```python
from build123d import *

# Parameters (mm, degrees)
F0_R     = 0.6
F1_DEPTH = 4


with BuildPart() as f1:
    # F0 (on Front) → F1 (new body)
    with BuildSketch(Plane.XZ):
        with BuildLine():
            ThreePointArc((8, 0), (9.478575, -1.518464), (10.999917, -0.042849))
            ThreePointArc((10.999917, -0.042849), (10.999979, -0.021425), (11, 0))
            ThreePointArc((11, 0), (0, 11), (-11, 0))
            ThreePointArc((-11, 0), (-1.5, 9.5), (8, 0))
        make_face()
        with Locations((9.5, 0)):
            Circle(F0_R, mode=Mode.SUBTRACT)
    extrude(amount=F1_DEPTH)


solid = f1.part
```
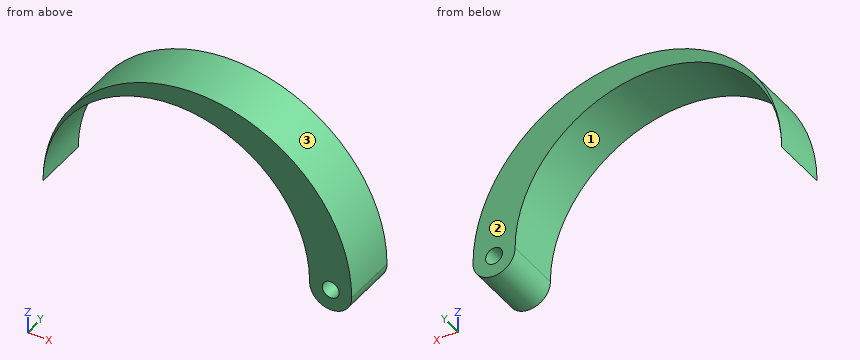
Work out the finished part from the listing and answer in its coordinate system (mm). Face numbers are marked on the shaded views. Round coordinates to 2 decimals unless told otherwise and drop trailing zeros. Order: outer loops, then holes, each group sorted by start corner. A loop starts at its lowest first (then second) coordinate and runs counter-clockwise, first axis right, second up.
Q1. A cutting plane is placed at C-C, the plane x = 9.5. Determine the outline of the cut face in (y, z), then the cut area to 3 significant figures.
Solution:
outline: (-4, -1.52) - (0, -1.52) - (0, -0.6) - (-4, -0.6) - close; (-4, 0.6) - (0, 0.6) - (0, 5.55) - (-4, 5.55) - close
area: 23.5 mm2
Q2. A cutting plane is placed at B-B, the plane y = -1.25. Determine the outline of the cut face in (x, z).
Solution:
outline: (-11, 0) arc R9.5 cw to (8, 0) arc R1.5 ccw to (11, -0.04) arc R11.19 ccw to (11, 0) arc R11 ccw to start; hole circle Ø1.2 at (9.5, 0)
Q3. A cutting plane is placed at D-D, the plane x = 2.25. Determine the outline of the cut face in (y, z).
Solution:
outline: (-4, 8.73) - (0, 8.73) - (0, 10.77) - (-4, 10.77) - close
Q4. A cutting plane is placed at A-A, the plane z = 7.25. Determine the outline of the cut face in (x, y), then the cut area to 3 significant figures.
Solution:
outline: (-8.27, -4) - (-7.64, -4) - (-7.64, 0) - (-8.27, 0) - close; (4.64, -4) - (8.27, -4) - (8.27, 0) - (4.64, 0) - close
area: 17.1 mm2
Q5. Given pin 1 Ø1.4 at (x, z) = (9.5, 0) entering from -Y; pin 2 Ø2 at (x, y) = (8, -3) entering from -Z; pin 3 Ø1.5 at (y, z) = (-2.5, 4) entering from +X; pin 4 Ø1 at (x, y) = (3, -3) entering from +Z, each flat-ended and moving along its own axis, determine where each tip first touches the part or whether it passes through.
Solution:
pin 1: stops at y = -4
pin 2: stops at z = -1.43
pin 3: stops at x = 10.51
pin 4: stops at z = 10.71
Q6. Find the intervals of material crossed by line 1 along X through (y, z) = (-0.85, 6.75); line 2 along Z through (x, y) = (9.5, -2.1); line 3 along X through (y, z) = (-0.45, 8.5), in increasing order.
Solution:
line 1: x = -8.69 to -8.18, 5.18 to 8.69
line 2: z = -1.52 to -0.6, 0.6 to 5.55
line 3: x = -6.98 to -5.74, 2.74 to 6.98
Q7. The mould has two halves that part along X. Classify the marked faces 1, 2 and 3: pulls with the +X half, pulls with the -X half, needs draft (parallel to the pull), parting line crosses it, or undercut.
Solution:
face 1: undercut
face 2: needs draft
face 3: parting line crosses it
